```python
from build123d import *

# Parameters (mm, degrees)
F0_R        = 6.35
F1_DEPTH    = 25.4
F2_SIZE     = 6.35
F3_W        = 19.05
F3_H        = 44.45
F4_DEPTH    = 76.2
F6_DEPTH    = 19.05
F8_DEPTH    = 25.4
F9_T1_DEPTH = 114.3


# Not quite as in the source:
# - a fillet or chamfer that OpenCascade refuses, or shapes differently, is made with other operations: its cross-section is extruded or revolved along the edge and cut away or added


with BuildPart() as f1:
    # F0 (on Top) → F1 (new body)
    with BuildSketch(Plane.XY):
        with BuildLine():
            Line((-4.9749455661, 42.822749579), (-74.8249455661, 42.822749579))
            ThreePointArc((-74.8249455661, 42.822749579), (-86.0502657174, 38.1730697303), (-90.6999455661, 26.947749579))
            Line((-90.6999455661, 26.947749579), (-90.6999455661, 1.547749579))
            ThreePointArc((-90.6999455661, 1.547749579), (-86.0502657174, -9.6775705724), (-74.8249455661, -14.327250421))
            Line((-74.8249455661, -14.327250421), (-4.9749455661, -14.327250421))
            ThreePointArc((-4.9749455661, -14.327250421), (6.2503745853, -9.6775705724), (10.9000544339, 1.547749579))
            Line((10.9000544339, 1.547749579), (10.9000544339, 26.947749579))
            ThreePointArc((10.9000544339, 26.947749579), (6.2503745853, 38.1730697303), (-4.9749455661, 42.822749579))
        make_face()
        with Locations((-74.8249455661, 1.547749579)):
            Circle(F0_R, mode=Mode.SUBTRACT)
        with Locations((-4.9749455661, 1.547749579)):
            Circle(F0_R, mode=Mode.SUBTRACT)
        with Locations((-74.8249455661, 26.947749579)):
            Circle(F0_R, mode=Mode.SUBTRACT)
        with Locations((-4.9749455661, 26.947749579)):
            Circle(F0_R, mode=Mode.SUBTRACT)
    extrude(amount=F1_DEPTH)

    # F2
    f2_edges = [f1.edges().sort_by_distance(p)[0] for p in [
        (6.250375, -9.677571, 25.4),
        (10.900054, 14.24775, 25.4),
        (6.250375, 38.17307, 25.4),
        (-39.899946, 42.82275, 25.4),
        (-86.050266, 38.17307, 25.4),
        (-90.699946, 14.24775, 25.4),
        (-86.050266, -9.677571, 25.4),
        (-39.899946, -14.32725, 25.4),
    ]]
    chamfer(f2_edges, length=F2_SIZE)

    # F3 (on face) → F4 (join)
    with BuildSketch(Plane.XY.offset(25.4)):
        with Locations((-55.7749455661, 14.247749579)):
            Rectangle(F3_W, F3_H)
    extrude(amount=F4_DEPTH)

    # F5 (on face) → F6 (cut, through all)
    with BuildSketch(Plane.YZ.offset(-46.2499455661)):
        with BuildLine():
            ThreePointArc((14.247749579, 41.6659471005), (25.4730697303, 46.3156269492), (30.122749579, 57.5409471005))
            ThreePointArc((30.122749579, 57.5409471005), (3.0224294276, 68.7662672519), (14.247749579, 41.6659471005))
        make_face()
    extrude(amount=-F6_DEPTH, mode=Mode.SUBTRACT)

    # F7 (on face) → F8 (cut)
    with BuildSketch(Plane.YZ.offset(-46.2499455661)):
        with BuildLine():
            ThreePointArc((-1.627250421, 57.5409471005), (14.247749579, 73.4159471005), (30.122749579, 57.5409471005))
            Line((30.122749579, 57.5409471005), (30.122749579, 101.6))
            Line((30.122749579, 101.6), (-1.627250421, 101.6))
            Line((-1.627250421, 101.6), (-1.627250421, 57.5409471005))
        make_face()
    extrude(amount=-F8_DEPTH, mode=Mode.SUBTRACT)

    # F9: fillet of radius 31.75 on 2 edges, made by hand

    # F9_s2 → F9_t1 (cut)
    with BuildSketch(Plane.YZ.offset(-112.9249455661)):
        with BuildLine():
            ThreePointArc((-7.977250421, 82.55), (-6.3479451342, 92.590231571), (-1.627250421, 101.6))
            Line((-1.627250421, 101.6), (-7.977250421, 101.6))
            Line((-7.977250421, 101.6), (-7.977250421, 82.55))
        make_face()
        with BuildLine():
            ThreePointArc((36.472749579, 82.55), (34.8434442921, 92.590231571), (30.122749579, 101.6))
            Line((30.122749579, 101.6), (36.472749579, 101.6))
            Line((36.472749579, 101.6), (36.472749579, 82.55))
        make_face()
    extrude(amount=F9_T1_DEPTH, mode=Mode.SUBTRACT)


solid = f1.part
```
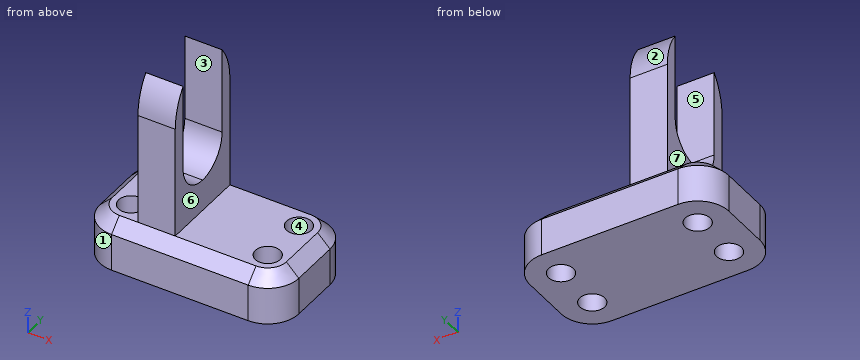
Here's how the part is built. I have some questions about the finished solid (model axes, mm). Face numbers are marked on the shaded views. A direction names the side the tool comes from. Give positions to 0.01 mm unless a question says otherwise; leave off trailing zeros. Order: outer loops, then holes, each group sorted by start corner. A loop starts at its lowest first (then second) coordinate and runs counter-clockwise, first axis right, second up. Notation, with made-up numbers: (85.5, 29.25) -> (131.5, 29.25) arc R16 ccw to (131.5, 60.25) -> close; hole circle Ø8 at (-3.5, 78). An arc over 180 degrees is marked (long way). Use CSV: the item, a comma, the result in double quotes. Start each with the question number.
Item 1: Suppose I cut it at A-A (z = 16). List the corners of the cut face in (x, y) for me (3 decimals).
Item 2: Thinking about a two-plate mould opening in Y: for the marked faces 1, 2 and 3, which applies, pulls with the +Y half, pulls with the -Y half, needs draft (parallel to the pull), parting line crosses it, or undercut?
Item 3: Suppose I cut it at B-B (z = 62.5). List the corners of the cut face in (x, y) for me.
Item 4: Suppose I cut it at C-C (x = -16.5). List the corners of the cut face in (y, z) for me.
Item 5: I'm going to push flat-ended pins straight in: P1, Ø14.5, axis at x = -4.97, y = 1.55, coming from the -Z side; P2, Ø21, axis at x = -55, z = 41.5, coming from the -Y side; P3, Ø22, axis at x = -26, y = 20, coming from the +Z side; P4, Ø15, axis at x = -55.5, z = 66, coming from the +Y side. Where does each tip first touch, or does it pass through?
Item 6: Suppose I cut it at D-D (y = 18.5). List the corners of the cut face in (x, z) for me, and give its area (3 significant figures).
Item 7: On a 3-axis mill with a long thin cutter (end or side, diameter ignored), from which of +Z, -Z, +X, -X, +Y, -Y can I reach the whole of each face in a straight line? I mean the marked faces 4, 5, 6 and 7. Say none if no direction works.
Item 8: If I drill on probe 1 along X at (y, z) = (1, 13); probe 2 along Y at (x, z) = (-71.5, 21); probe 3 along X at (y, z) = (5, 21.5), over which ranges is the centre line in solid material (lowest first)? Write a range as [from, to].
Answer block:
1,outline,"(-90.7, 1.548) arc R15.875 ccw to (-74.825, -14.327) -> (-4.975, -14.327) arc R15.875 ccw to (10.9, 1.548) -> (10.9, 26.948) arc R15.875 ccw to (-4.975, 42.823) -> (-74.825, 42.823) arc R15.875 ccw to (-90.7, 26.948) -> close; hole circle Ø12.7 at (-74.825, 1.548); hole circle Ø12.7 at (-74.825, 26.948); hole circle Ø12.7 at (-4.975, 1.548); hole circle Ø12.7 at (-4.975, 26.948)"
2,face 1,"pulls with the -Y half"
2,face 2,"pulls with the +Y half"
2,face 3,"undercut"
3,outline,"(-65.3, -7.98) -> (-46.25, -7.98) -> (-46.25, -1.63) -> (-65.3, -1.63) -> close; (-65.3, 30.12) -> (-46.25, 30.12) -> (-46.25, 36.47) -> (-65.3, 36.47) -> close"
4,outline,"(-14.33, 0) -> (42.82, 0) -> (42.82, 19.05) -> (36.47, 25.4) -> (-7.98, 25.4) -> (-14.33, 19.05) -> close"
5,P1,"stops at z = 0"
5,P2,"stops at y = -7.98"
5,P3,"stops at z = 25.4"
5,P4,"stops at y = 36.47"
6,outline,"(-90.7, 0) -> (10.9, 0) -> (10.9, 19.05) -> (4.55, 25.4) -> (-46.25, 25.4) -> (-46.25, 42.25) -> (-65.3, 42.25) -> (-65.3, 25.4) -> (-84.35, 25.4) -> (-90.7, 19.05) -> close"
6,area,"2,860 mm^2"
7,face 4,"+Z, -Z"
7,face 5,"+Z, +X, -X"
7,face 6,"+Z, +X, +Y, -Y"
7,face 7,"+Z, -X, +Y, -Y"
8,probe 1,"x = [-90.69, -81.15], [-68.5, -11.3], [1.35, 10.89]"
8,probe 2,"y = [-12.38, -3.86], [6.96, 21.54], [32.36, 40.87]"
8,probe 3,"x = [-88.25, -80.15], [-69.5, -10.3], [0.35, 8.45]"
